Study the drawing (mm; zero at the part's minimum x, y, z) and answer. A direction names the side the tool comes from. Give positions to 0.01 mm unless a question says otherwise; leave off trailing zeros. Write each loop counter-clockwise with the first axis right and the second up, starting at its lowest first coordinate (ties: lowest second). Pieces come first, ordered by that corner, then holes. Notation, with made-up numbers: M 33.5,1 L 73.5,1 A25 cw 73.5,23 Z; hole C 75.25,14 d9. An arc over 180 degrees is marked long. Use a Markdown table: item, result. Add a question column.
Item 1: A cutting plane is placed at B-B on y = 5. Determine the outline of the cut face in (x, z).
Item 2: Consider probe 1 along Z at (x, y) = (3, 4.5); probe 2 along X at (y, z) = (0.75, 4); probe 3 along Y at (x, z) = (0.5, 4). Determine where each line is inside the solid, lowest interval first. Write a range as [from, to].
Item 3: A cutting plane is placed at A-A on x = 6. Determine the outline of the cut face in (y, z), then the cut area to 3 significant figures.
Item 4: For the marked faces 1 and 2, determine the directions among +Z, -Z, +X, -X, +Y, -Y from which every point of the face is accessible in a straight line to the end or side of a thin tool.
Item 5: A cutting plane is placed at C-C on z = 9.25. Determine the outline of the cut face in (x, y), then the cut area to 3 significant figures.
Item 6: A cutting plane is placed at D-D on y = 2.75. Determine the outline of the cut face in (x, z).
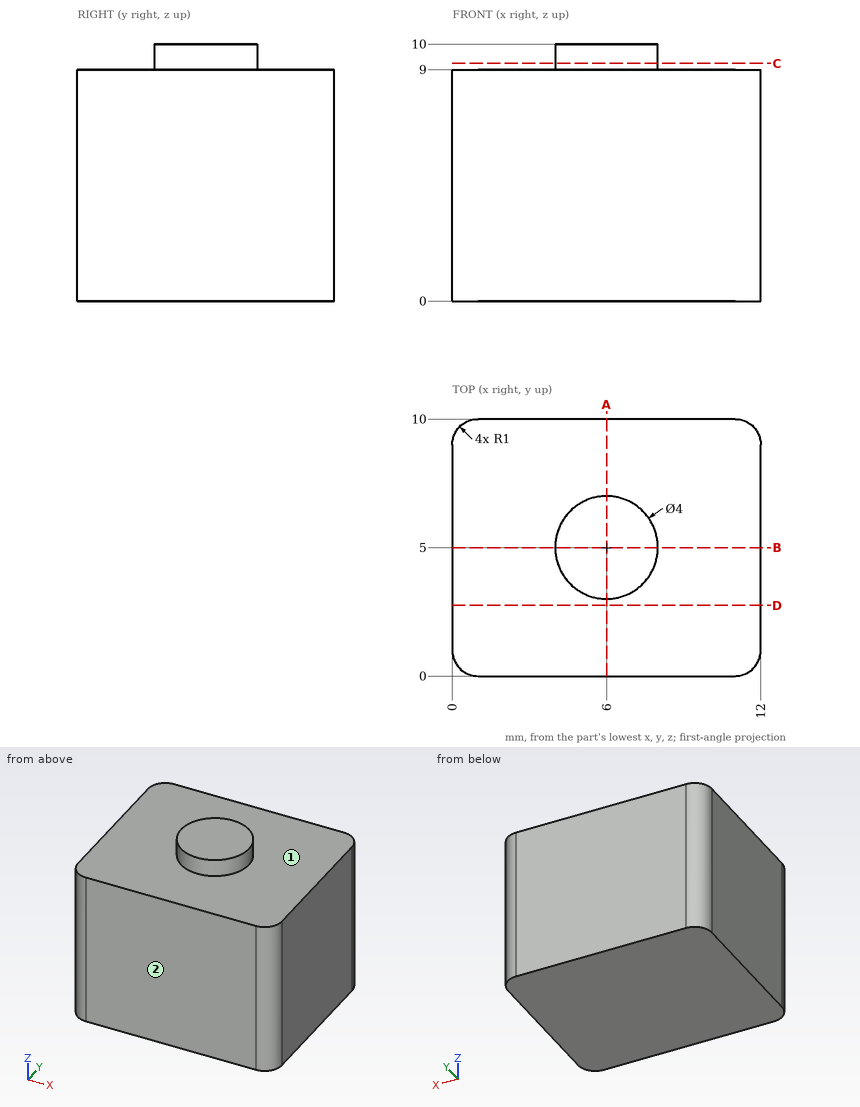
Filled in:
| question | item | result |
|---|---|---|
| 1 | outline | M 0,0 L 12,0 L 12,9 L 8,9 L 8,10 L 4,10 L 4,9 L 0,9 Z |
| 2 | probe 1 | [0, 9] |
| 2 | probe 2 | [0.03, 11.97] |
| 2 | probe 3 | [0.13, 9.87] |
| 3 | outline | M 0,0 L 10,0 L 10,9 L 7,9 L 7,10 L 3,10 L 3,9 L 0,9 Z |
| 3 | area | 94.0 mm² |
| 4 | face 1 | +Z |
| 4 | face 2 | +Z, -Z, +X, -X, -Y |
| 5 | outline | C 6,5 d4 |
| 5 | area | 12.6 mm² |
| 6 | outline | M 0,0 L 12,0 L 12,9 L 0,9 Z |
